```python
from build123d import *

# Parameters (mm, degrees)
F1_DEPTH = 426
F3_DEPTH = 4
F4_R     = 2


# Not quite as in the source:
# - a feature names something its author has since deleted; it is built from what else it names


with BuildPart() as f1:
    # F0 (on Top) → F1 (new body)
    with BuildSketch(Plane.XY):
        Polygon((495, 0), (0, 0), (0, -343), (200, -343), (200, -1053), (204, -1053), (204, -339), (4, -339), (4, -4), (491, -4), (491, -1053), (495, -1053), align=None)
    extrude(amount=F1_DEPTH)

    # F2 (on Top) → F3 (join)
    with BuildSketch(Plane.XY):
        Polygon((0, -343), (200, -343), (199.9874711037, -1053), (495, -1053), (495, 0), (0, 0), align=None)
    extrude(amount=-F3_DEPTH)

    # F4
    f4_edges = [f1.edges().sort_by_distance(p)[0] for p in [
        (100, -343, -4),
        (0, -171.5, -4),
        (247.5, 0, -4),
        (0, -343, 211),
        (0, 0, 211),
        (495, 0, 211),
        (199.993736, -698, -4),
        (495, -526.5, -4),
    ]]
    fillet(f4_edges, radius=F4_R)


solid = f1.part
```
The listing builds one solid part. Answer for the finished solid, in the listing's coordinates (mm). A direction names the side the tool comes from. Round coordinates to 2 decimals unless told otherwise and drop trailing zeros. Order: outer loops, then holes, each group sorted by start corner. A loop starts at its lowest first (then second) coordinate and runs counter-clockwise, first axis right, second up. Notation, with made-up numbers: (54, 54) -> (108, 54) arc R5 cw to (108, 58) -> close; hole circle Ø2 at (80.25, 8.25). An arc over 180 degrees is marked (long way). Answer as CSV lines item,"result". Start each with the question number.
(1) The part is cut by section C-C (z = 373). Determine the outline of the cut face in (x, y).
(2) The part is cut by section D-D (x = 127.5). Determine the outline of the cut face in (y, z).
(3) Flat-ended cylindrical pins translate along their axes: pin 1 Ø2 at (x, y) = (416, -344) entering from +Z; pin 2 Ø2 at (y, z) = (-636.5, 254.5) entering from -X; pin 3 Ø6 at (x, z) = (65.5, 62) entering from -Y. Find the tip coordinate at first contact, or state that the pin passes through.
(4) The part is cut by section B-B (x = 307). Determine the outline of the cut face in (y, z), then the cut area to 3 significant figures.
(5) For a pull along X with two mould halves and no side action, classify faces 4 (the face through (200, -693, 210)), 5 (the face through (298, -405, 0)), 6 (the face through (100, -343, 215)) as +X half, -X half, draft (parallel to the pull), parting line (faces both ways), or undercut.
(6) Find the intervals of material crossed by probe 1 along Y at (x, z) = (154, 318); probe 2 along X at (y, z) = (-126, 183.5); probe 3 along X at (y, z) = (-901.5, 218), in increasing order. Write a range as from..to.
(7) The part is cut by section A-A (y = -303). Determine the outline of the cut face in (x, z).
(8) A tool of negligible diameter and unlimited length cuts with its end or side. For faces 1 (the face through (204, -701, 210)), 2 (the face through (0, -169, 215)), 3 (the face through (105, -339, 210)), from which of +Z, -Z, +X, -X, +Y, -Y can it reach the whole face along a straight path? Write none if from no direction.
Evaluation:
1,outline,"(0, -341) arc R2 ccw to (2, -343) -> (200, -343) -> (200, -1053) -> (204, -1053) -> (204, -339) -> (4, -339) -> (4, -4) -> (491, -4) -> (491, -1053) -> (495, -1053) -> (495, -2) arc R2 ccw to (493, 0) -> (2, 0) arc R2 ccw to (0, -2) -> close"
2,outline,"(-343, -2) arc R2 ccw to (-341, -4) -> (-2, -4) arc R2 ccw to (0, -2) -> (0, 426) -> (-4, 426) -> (-4, 0) -> (-339, 0) -> (-339, 426) -> (-343, 426) -> close"
3,pin 1,"z = 0"
3,pin 2,"x = 200"
3,pin 3,"y = -343"
4,outline,"(-1053, -4) -> (-2, -4) arc R2 ccw to (0, -2) -> (0, 426) -> (-4, 426) -> (-4, 0) -> (-1053, 0) -> close"
4,area,"5,920 mm²"
5,face 4,"-X half"
5,face 5,"undercut"
5,face 6,"draft"
6,probe 1,"-343..-339, -4..0"
6,probe 2,"0..4, 491..495"
6,probe 3,"200..204, 491..495"
7,outline,"(0, -2) arc R2 ccw to (2, -4) -> (493, -4) arc R2 ccw to (495, -2) -> (495, 426) -> (491, 426) -> (491, 0) -> (4, 0) -> (4, 426) -> (0, 426) -> close"
8,face 1,"+Z, -Y"
8,face 2,"+Z, -Z, -X, +Y, -Y"
8,face 3,"+Z"
